Could you check a few things on this model? Use its own coordinates, in mm. Round coordinates to 2 decimals unless told otherwise and drop trailing zeros. Write each loop counter-clockwise with the first axis right and the second up, starting at its lowest first coordinate (ties: lowest second). Pieces come first, ordered by that corner, then holes.
```python
from build123d import *

# Parameters (mm, degrees)
BOSS_EXTRUDE1_DEPTH = 3
SKETCH2_R           = 2.55
SKETCH2_R_2         = 3.6
CUT_EXTRUDE1_DEPTH  = 47.412552181


with BuildPart() as part:
    # Sketch1 → Boss-Extrude1 (new body)
    with BuildSketch(Plane(origin=(0, 0, 0), x_dir=(1, 0, 0), z_dir=(0, 1, 0))):
        with BuildLine():
            Line((-29.75, 32.75), (29.75, 32.75))
            ThreePointArc((29.75, 32.75), (31.871320344, 31.871320344), (32.75, 29.75))
            Line((32.75, 29.75), (32.75, -29.75))
            ThreePointArc((32.75, -29.75), (31.871320344, -31.871320344), (29.75, -32.75))
            Line((29.75, -32.75), (-29.75, -32.75))
            ThreePointArc((-29.75, -32.75), (-31.871320344, -31.871320344), (-32.75, -29.75))
            Line((-32.75, -29.75), (-32.75, 29.75))
            ThreePointArc((-32.75, 29.75), (-31.871320344, 31.871320344), (-29.75, 32.75))
        make_face()
    extrude(amount=BOSS_EXTRUDE1_DEPTH)

    # Sketch2 → Cut-Extrude1 (cut, through all)
    with BuildSketch(Plane(origin=(0, 3, 0), x_dir=(1, 0, 0), z_dir=(0, 1, 0))):
        with Locations(Location((0, 0, 0), (0, 0, 270))):
            Circle(SKETCH2_R)
        with Locations(Location((-20, -20, 0), (0, 0, 270))):
            Circle(SKETCH2_R_2)
        with Locations(Location((-20, -10, 0), (0, 0, 270))):
            Circle(SKETCH2_R)
        with Locations(Location((-20, 0, 0), (0, 0, 270))):
            Circle(SKETCH2_R_2)
        with Locations(Location((-20, 10, 0), (0, 0, 270))):
            Circle(SKETCH2_R)
        with Locations(Location((-20, 20, 0), (0, 0, 270))):
            Circle(SKETCH2_R_2)
        with Locations(Location((-10, 0, 0), (0, 0, 270))):
            Circle(SKETCH2_R)
        with Locations(Location((10, 0, 0), (0, 0, 270))):
            Circle(SKETCH2_R)
        with Locations(Location((20, 0, 0), (0, 0, 270))):
            Circle(SKETCH2_R)
        with Locations(Location((0, -10, 0), (0, 0, 270))):
            Circle(SKETCH2_R)
        with Locations(Location((0, 10, 0), (0, 0, 270))):
            Circle(SKETCH2_R)
        with Locations(Location((20, -10, 0), (0, 0, 270))):
            Circle(SKETCH2_R)
        with Locations(Location((20, 10, 0), (0, 0, 270))):
            Circle(SKETCH2_R)
        with Locations(Location((20, 20, 0), (0, 0, 270))):
            Circle(SKETCH2_R)
        with Locations(Location((20, -20, 0), (0, 0, 270))):
            Circle(SKETCH2_R)
        with BuildLine():
            Line((-23.4, 29.2), (-16.6, 29.2))
            ThreePointArc((-16.6, 29.2), (-15.1, 27.7), (-16.6, 26.2))
            Line((-16.6, 26.2), (-23.4, 26.2))
            ThreePointArc((-23.4, 26.2), (-24.9, 27.7), (-23.4, 29.2))
        make_face()
        with BuildLine():
            Line((-3.4, 29.2), (3.4, 29.2))
            ThreePointArc((3.4, 29.2), (4.9, 27.7), (3.4, 26.2))
            Line((3.4, 26.2), (-3.4, 26.2))
            ThreePointArc((-3.4, 26.2), (-4.9, 27.7), (-3.4, 29.2))
        make_face()
        with BuildLine():
            Line((16.6, 29.2), (23.4, 29.2))
            ThreePointArc((23.4, 29.2), (24.9, 27.7), (23.4, 26.2))
            Line((23.4, 26.2), (16.6, 26.2))
            ThreePointArc((16.6, 26.2), (15.1, 27.7), (16.6, 29.2))
        make_face()
        with BuildLine():
            Line((-3.4, -26.2), (3.4, -26.2))
            ThreePointArc((3.4, -26.2), (4.9, -27.7), (3.4, -29.2))
            Line((3.4, -29.2), (-3.4, -29.2))
            ThreePointArc((-3.4, -29.2), (-4.9, -27.7), (-3.4, -26.2))
        make_face()
        with BuildLine():
            Line((16.6, -26.2), (23.4, -26.2))
            ThreePointArc((23.4, -26.2), (24.9, -27.7), (23.4, -29.2))
            Line((23.4, -29.2), (16.6, -29.2))
            ThreePointArc((16.6, -29.2), (15.1, -27.7), (16.6, -26.2))
        make_face()
        with BuildLine():
            Line((-23.4, -26.2), (-16.6, -26.2))
            ThreePointArc((-16.6, -26.2), (-15.1, -27.7), (-16.6, -29.2))
            Line((-16.6, -29.2), (-23.4, -29.2))
            ThreePointArc((-23.4, -29.2), (-24.9, -27.7), (-23.4, -26.2))
        make_face()
        with BuildLine():
            Line((-10, 22.5), (10, 22.5))
            ThreePointArc((10, 22.5), (12.5, 20), (10, 17.5))
            Line((10, 17.5), (-10, 17.5))
            ThreePointArc((-10, 17.5), (-12.5, 20), (-10, 22.5))
        make_face()
        with BuildLine():
            Line((10, -17.5), (-10, -17.5))
            ThreePointArc((-10, -17.5), (-12.5, -20), (-10, -22.5))
            Line((-10, -22.5), (10, -22.5))
            ThreePointArc((10, -22.5), (12.5, -20), (10, -17.5))
        make_face()
    extrude(amount=-CUT_EXTRUDE1_DEPTH, mode=Mode.SUBTRACT)


solid = part.part
```
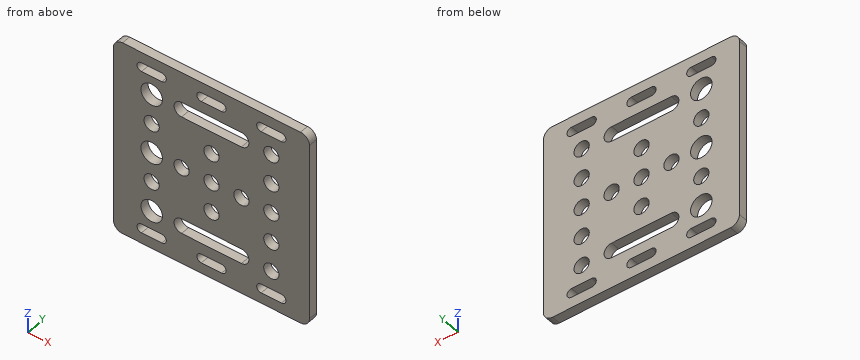
Q1. If I drill on L1, parallel to X at y = 2.25, z = -10; L2, parallel to X at y = 1.95, z = 0.5; L3, parallel to X at y = 1.4, z = -9, over which ranges is the centre line in solid material (lowest first)?
Q2. Imagine slicing it at B-B, the plane z = 27.7. Write out the boundary of the cut face in (x, y).
Q3. Imagine slicing it at C-C, the plane x = 1.5. Count the separate pieces of the cut face and the enclosed holes in it, then the cut area to 3 significant figures.
Q4. Imagine slicing it at A-A, the plane z = 0. Write out the boundary of the cut face in (x, y), then the cut area to 3 significant figures.
Results found:
1. L1: x = -32.75 to -22.55, -17.45 to -2.55, 2.55 to 17.45, 22.55 to 32.75
1. L2: x = -32.75 to -23.57, -16.43 to -12.5, -7.5 to -2.5, 2.5 to 7.5, 12.5 to 17.5, 22.5 to 32.75
1. L3: x = -32.75 to -22.35, -17.65 to -2.35, 2.35 to 17.65, 22.35 to 32.75
2. outline: (-32.75, 0) - (-24.9, 0) - (-24.9, 3) - (-32.75, 3) - close; (-15.1, 0) - (-4.9, 0) - (-4.9, 3) - (-15.1, 3) - close; (4.9, 0) - (15.1, 0) - (15.1, 3) - (4.9, 3) - close; (24.9, 0) - (32.75, 0) - (32.75, 3) - (24.9, 3) - close
3. separate pieces: 8
3. enclosed holes: 0
3. area: 111 mm2
4. outline: (-32.75, 0) - (-23.6, 0) - (-23.6, 3) - (-32.75, 3) - close; (-16.4, 0) - (-12.55, 0) - (-12.55, 3) - (-16.4, 3) - close; (-7.45, 0) - (-2.55, 0) - (-2.55, 3) - (-7.45, 3) - close; (2.55, 0) - (7.45, 0) - (7.45, 3) - (2.55, 3) - close; (12.55, 0) - (17.45, 0) - (17.45, 3) - (12.55, 3) - close; (22.55, 0) - (32.75, 0) - (32.75, 3) - (22.55, 3) - close
4. area: 114 mm2
